The model under review builds one solid part; all positions refer to its coordinate system, in mm. Face numbers are marked on the shaded views. A direction names the side the tool comes from. Round coordinates to 2 decimals unless told otherwise and drop trailing zeros. Loops run counter-clockwise (first coordinate to the right, second up) from the corner with the lowest first, then second, coordinate; pieces in that order, holes last. Notation, with made-up numbers: M 62,77 L 114,77 A25 cw 114,91 Z; hole C 58.5,-35 d4. An arc over 180 degrees is marked long. Answer as a JSON object with one key per item and string values. Group by question number.
Item 1: To check wall thickness, follow line 1 (Y direction, x = 0.4, z = 0.75); line 2 (Y direction, x = 2.05, z = -0.2); line 3 (Z direction, x = -0.6, y = -19.5). State the ranges of each line that lie inside material, in increasing order.
Item 2: Consider section A-A (x = 0). Give the boundary of the cut face in (y, z) (3 decimals), and give its area (3 significant figures).
Item 3: Insertion check: P1, Ø1, axis at x = 0.5, y = -19.5, coming from the -Z side; P2, Ø2, axis at y = -14, z = -2, coming from the -X side; P3, Ø1.8, axis at x = 0, z = 0, coming from the +Y side. Each pin has a flat end and moves straight along its axis. Give the tip position at first contact, or say it passes through.
Item 4: Tool access review of the marked faces 1 and 2: name each direction out of +Z, -Z, +X, -X, +Y, -Y from which nothing blocks a thin tool from reaching the whole face with its end or side.
Item 5: Consider section B-B (y = -3). Give the boundary of the cut face in (x, z), and give its area (3 significant figures).
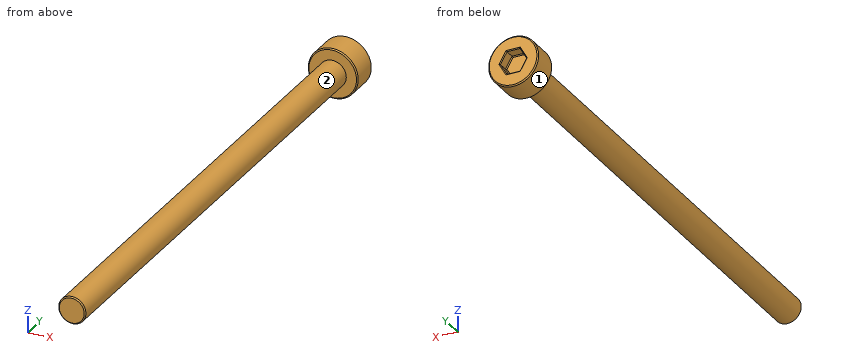
```python
from build123d import *

# Parameters (mm, degrees)
SKETCH1_R           = 2.75
BOSS_EXTRUDE1_DEPTH = 3
SKETCH2_R           = 1.5
BOSS_EXTRUDE2_DEPTH = 55
CHAMFER1_SIZE       = 0.125
CHAMFER2_SIZE       = 0.125
CUT_EXTRUDE1_DEPTH  = 1.25
CHAMFER3_SIZE       = 0.1
CHAMFER4_SIZE       = 0.1


with BuildPart() as part:
    # Sketch1 → Boss-Extrude1 (new body)
    with BuildSketch(Plane(origin=(0, 0, 0), x_dir=(1, 0, 0), z_dir=(0, 1, 0))):
        with Locations(Location((0, 0, 0), (0, 0, 270))):
            Circle(SKETCH1_R)
    extrude(amount=BOSS_EXTRUDE1_DEPTH)

    # Sketch2 → Boss-Extrude2 (add)
    with BuildSketch(Plane(origin=(0, 0, 0), x_dir=(-1, 0, 0), z_dir=(0, -1, 0))):
        with Locations(Location((0, 0, 0), (0, 0, 90))):
            Circle(SKETCH2_R)
    extrude(amount=BOSS_EXTRUDE2_DEPTH)

    # Chamfer1
    chamfer1_edges = [part.edges().sort_by_distance(p)[0] for p in [
        (0, 0, -2.75),
        (0, 3, -2.75),
    ]]
    chamfer(chamfer1_edges, length=CHAMFER1_SIZE)

    # Chamfer2
    chamfer2_edges = [part.edges().sort_by_distance(p)[0] for p in [
        (0, -55, 1.5),
    ]]
    chamfer(chamfer2_edges, length=CHAMFER2_SIZE)

    # Sketch3 → Cut-Extrude1 (cut)
    with BuildSketch(Plane(origin=(0, 3, 0), x_dir=(1, 0, 0), z_dir=(0, 1, 0))):
        Polygon((1.443375673, 0), (0.721687836, 1.25), (-0.721687836, 1.25), (-1.443375673, 0), (-0.721687836, -1.25), (0.721687836, -1.25), align=None)
    extrude(amount=-CUT_EXTRUDE1_DEPTH, mode=Mode.SUBTRACT)

    # Chamfer3
    chamfer3_edges = [part.edges().sort_by_distance(p)[0] for p in [
        (1.082531755, 3, 0.625),
        (1.082531755, 3, -0.625),
        (0, 3, -1.25),
        (-1.082531755, 3, -0.625),
        (-1.082531755, 3, 0.625),
        (0, 3, 1.25),
    ]]
    chamfer(chamfer3_edges, length=CHAMFER3_SIZE)

    # Chamfer4
    chamfer4_edges = [part.edges().sort_by_distance(p)[0] for p in [
        (1.082531755, 1.75, 0.625),
        (0, 1.75, 1.25),
        (-1.082531755, 1.75, 0.625),
        (-1.082531755, 1.75, -0.625),
        (0, 1.75, -1.25),
        (1.082531755, 1.75, -0.625),
    ]]
    chamfer(chamfer4_edges, length=CHAMFER4_SIZE)


solid = part.part
```
Geometry results:
{
 "1": {"line 1": "y = -55 to 1.75", "line 2": "y = 0 to 3", "line 3": "z = -1.37 to 1.37"},
 "2": {"outline": "M -55,-1.375 L -54.875,-1.5 L 0,-1.5 L 0,-2.625 L 0.125,-2.75 L 2.875,-2.75 L 3,-2.625 L 3,-1.35 L 2.9,-1.25 L 1.85,-1.25 L 1.75,-1.15 L 1.75,1.15 L 1.85,1.25 L 2.9,1.25 L 3,1.35 L 3,2.625 L 2.875,2.75 L 0.125,2.75 L 0,2.625 L 0,1.5 L -54.875,1.5 L -55,1.375 Z", "area": "178 mm^2"},
 "3": {"P1": "stops at z = -1.5", "P2": "stops at x = -1.12", "P3": "stops at y = 1.75"},
 "4": {"face 1": "+Y, -Y", "face 2": "-Y"},
 "5": {"outline": "C 0,0 d3", "area": "7.07 mm^2"}
}
